Answer from the drawing. Dimensions are ordinates in mm from the lowest x, y and z of the part. A direction names the side the tool comes from. Coordinates: 2 decimals unless noted, no trailing zeros. Order: outer loops, then holes, each group sorted by start corner. A loop starts at its lowest first (then second) coordinate and runs counter-clockwise, first axis right, second up. Notation, with made-up numbers: (75.25, 44.5) -> (130.25, 44.5) arc R23 ccw to (130.25, 75.5) -> close; hole circle Ø9 at (66, 51.5). An arc over 180 degrees is marked (long way). Answer in a Markdown table with one row per item.
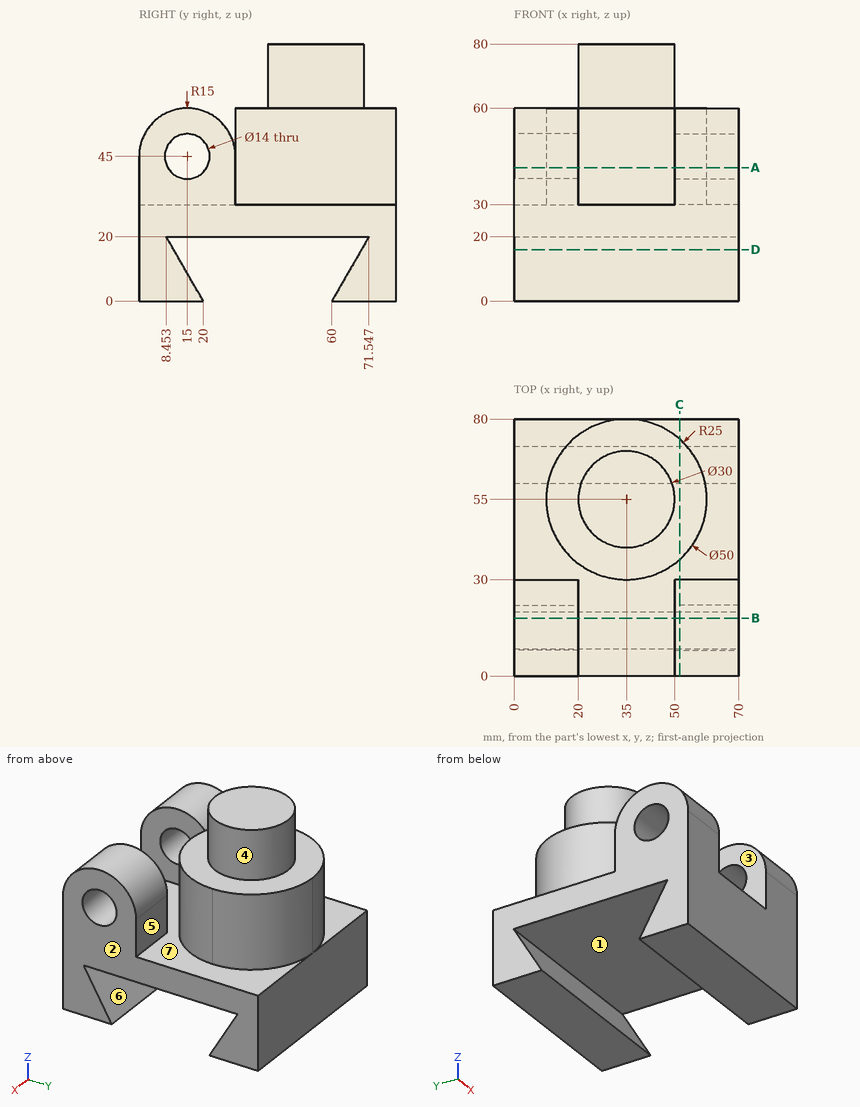
Q1. Given pin 1 (1.5 mm diameter, centred on x = 12.5, z = 34.5, fed in from +Y); pin 2 (11 mm diameter, centred on y = 15, z = 45, fed in from -X); pin 3 (22.5 mm diameter, centred on y = 15, z = 45, fed in from +X); pin 4 (12 mm diameter, centred on x = 13.5, z = 41, fed in from +Y) (3 decimals), each flat-ended and moving along its own axis, determine where each tip first touches the part or whether it passes through.
Outcome:
| item | result |
|---|---|
| pin 1 | y = 67.33 |
| pin 2 | through |
| pin 3 | x = 70 |
| pin 4 | y = 74.615 |
Q2. The part is cut by section D-D (z = 16). Write down the section's boundary in (x, y).
Outcome:
| item | result |
|---|---|
| outline | (0, 0) -> (70, 0) -> (70, 10.76) -> (0, 10.76) -> close; (0, 69.24) -> (70, 69.24) -> (70, 80) -> (0, 80) -> close |
Q3. The part is cut by section B-B (y = 18). Write down the section's boundary in (x, z).
Outcome:
| item | result |
|---|---|
| outline | (0, 0) -> (70, 0) -> (70, 3.46) -> (0, 3.46) -> close; (0, 20) -> (70, 20) -> (70, 38.68) -> (50, 38.68) -> (50, 30) -> (20, 30) -> (20, 38.68) -> (0, 38.68) -> close; (0, 51.32) -> (20, 51.32) -> (20, 59.7) -> (0, 59.7) -> close; (50, 51.32) -> (70, 51.32) -> (70, 59.7) -> (50, 59.7) -> close |
Q4. For the marked faces 5, 6 and 7, determine the directions among +Z, -Z, +X, -X, +Y, -Y from which every point of the face is accessible in a straight line to the end or side of a thin tool.
Outcome:
| item | result |
|---|---|
| face 5 | +Z, +X |
| face 6 | +X, -X |
| face 7 | +Z |
Q5. The part is cut by section C-C (x = 51.5). Write down the section's boundary in (y, z).
Outcome:
| item | result |
|---|---|
| outline | (0, 0) -> (20, 0) -> (8.45, 20) -> (71.55, 20) -> (60, 0) -> (80, 0) -> (80, 30) -> (73.78, 30) -> (73.78, 60) -> (36.22, 60) -> (36.22, 30) -> (30, 30) -> (30, 45) arc R15 ccw to (0, 45) -> close; hole circle Ø14 at (15, 45) |
Q6. Consider line 1 (X direction, y = 9, z = 50); line 2 (Z direction, x = 11, y = 15); line 3 (X direction, y = 35, z = 47). Determine where each line is inside the solid, lowest interval first.
Outcome:
| item | result |
|---|---|
| line 1 | 0 to 20, 50 to 70 |
| line 2 | 0 to 8.66, 20 to 38, 52 to 60 |
| line 3 | 20 to 50 |
Q7. The part is cut by section A-A (z = 41.5). Write down the section's boundary in (x, y).
Outcome:
| item | result |
|---|---|
| outline | (0, 0) -> (20, 0) -> (20, 8.94) -> (0, 8.94) -> close; (0, 21.06) -> (20, 21.06) -> (20, 30) -> (0, 30) -> close; circle Ø50 at (35, 55); (50, 0) -> (70, 0) -> (70, 8.94) -> (50, 8.94) -> close; (50, 21.06) -> (70, 21.06) -> (70, 30) -> (50, 30) -> close |
Q8. For a pull along X with two mould halves and no side action, classify the marked faces 1, 2, 3 and 4 as pulls with the +X half, pulls with the -X half, needs draft (parallel to the pull), parting line crosses it, or undercut.
Outcome:
| item | result |
|---|---|
| face 1 | needs draft |
| face 2 | pulls with the +X half |
| face 3 | undercut |
| face 4 | parting line crosses it |
